The model under review builds one solid part; all positions refer to its coordinate system, in mm. Face numbers are marked on the shaded views. A direction names the side the tool comes from. Round coordinates to 2 decimals unless told otherwise and drop trailing zeros. Loops run counter-clockwise (first coordinate to the right, second up) from the corner with the lowest first, then second, coordinate; pieces in that order, holes last. Notation, with made-up numbers: M 16.25,29.5 L 74.25,29.5 A19 cw 74.25,55.5 Z; hole C 84.25,62 d6. An arc over 180 degrees is marked long. Use a Markdown table: item, result. Add a question column.
```python
from build123d import *

# Parameters (mm, degrees)
F0_R      = 9.525
F1_DEPTH  = 31.75
F2_R      = 9.99744
F3_DEPTH  = 28.575
F4_R      = 11.1125
F5_DEPTH  = 45.0342
F6_R      = 10.7696
F7_DEPTH  = 82.169
F8_R      = 9.99744
F9_DEPTH  = 41.275
F10_R     = 9.525
F11_DEPTH = 76.5302
F12_R     = 12.5854341712
F13_DEPTH = 3.175
F14_DEPTH = 3.175


with BuildPart() as f1:
    # F0 (on Right) → F1 (new body)
    with BuildSketch(Plane.YZ):
        Circle(F0_R)
    extrude(amount=F1_DEPTH)

    # F2 (on face) → F3 (join)
    with BuildSketch(Plane.YZ.offset(31.75)):
        Circle(F2_R)
    extrude(amount=F3_DEPTH)

    # F4 (on face) → F5 (join)
    with BuildSketch(Plane.YZ.offset(60.325)):
        Circle(F4_R)
    extrude(amount=F5_DEPTH)

    # F6 (on face) → F7 (join)
    with BuildSketch(Plane.YZ.offset(105.3592)):
        Circle(F6_R)
    extrude(amount=F7_DEPTH)

    # F8 (on face) → F9 (join)
    with BuildSketch(Plane.YZ.offset(187.5282)):
        Circle(F8_R)
    extrude(amount=F9_DEPTH)

    # F10 (on face) → F11 (join)
    with BuildSketch(Plane.YZ.offset(228.8032)):
        Circle(F10_R)
    extrude(amount=F11_DEPTH)

    # F12 (on Top) → F13 (cut)
    with BuildSketch(Plane.XY):
        with Locations((77.320471406, -12.4823525548)):
            Circle(F12_R)
    extrude(amount=F13_DEPTH, mode=Mode.SUBTRACT)

    # F14 (cut): a face of the model
    f14_faces = [f1.faces().sort_by_distance(p)[0] for p in [
        (77.320471406, -6.3933996549, 0),
    ]]
    extrude(f14_faces, amount=-F14_DEPTH, mode=Mode.SUBTRACT)


solid = f1.part
```
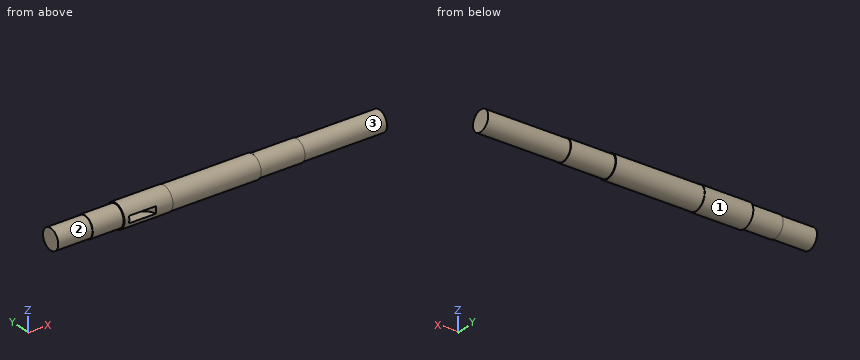
(1) Insertion check: pin 1 Ø1 at (y, z) = (8.5, 6.5) entering from +X; pin 2 Ø5.5 at (x, y) = (80.5, -5.5) entering from -Z; pin 3 Ø3 at (x, y) = (254, -7.5) entering from -Z; pin 4 Ø12 at (x, y) = (80, -5.5) entering from +Z. Each pin has a flat end and moves straight along its axis. Give the tip position at first contact, or say it passes through.
(2) For the marked faces 1, 2 and 3, list the 3-axis set-ups (+Z, -Z, +X, -X, +Y, -Y) from which the entire face can be reached by the end or side of a thin tool; tool diameter is ignored.
(3) Consider section B-B, the plane y = 3.75. Give the boundary of the cut face in (x, z) (3 decimals).
(4) Consider section D-D, the plane x = 163. Give the boundary of the cut face in (y, z).
(5) Consider section C-C, the plane x = 285.5. Give the boundary of the cut face in (y, z) (3 decimals).
(6) To check wall thickness, follow probe 1 along Y at (x, z) = (246.5, -1); probe 2 along X at (y, z) = (3.5, -9); probe 3 along Z at (x, y) = (184, 5). State the ranges of each line that lie inside material, in increasing order.
Found:
| question | item | result |
|---|---|---|
| 1 | pin 1 | stops at x = 187.53 |
| 1 | pin 2 | stops at z = -10.77 |
| 1 | pin 3 | stops at z = -7.4 |
| 1 | pin 4 | stops at z = 11.11 |
| 2 | face 1 | +X, -X |
| 2 | face 2 | -X |
| 2 | face 3 | +X |
| 3 | outline | M 0,-8.756 L 31.75,-8.756 L 31.75,-9.267 L 60.325,-9.267 L 60.325,-10.461 L 105.359,-10.461 L 105.359,-10.096 L 187.528,-10.096 L 187.528,-9.267 L 228.803,-9.267 L 228.803,-8.756 L 305.333,-8.756 L 305.333,8.756 L 228.803,8.756 L 228.803,9.267 L 187.528,9.267 L 187.528,10.096 L 105.359,10.096 L 105.359,10.461 L 60.325,10.461 L 60.325,9.267 L 31.75,9.267 L 31.75,8.756 L 0,8.756 Z |
| 4 | outline | C 0,0 d21.54 |
| 5 | outline | C 0,0 d19.05 |
| 6 | probe 1 | y = -9.47 to 9.47 |
| 6 | probe 2 | x = 31.75 to 228.8 |
| 6 | probe 3 | z = -9.54 to 9.54 |
